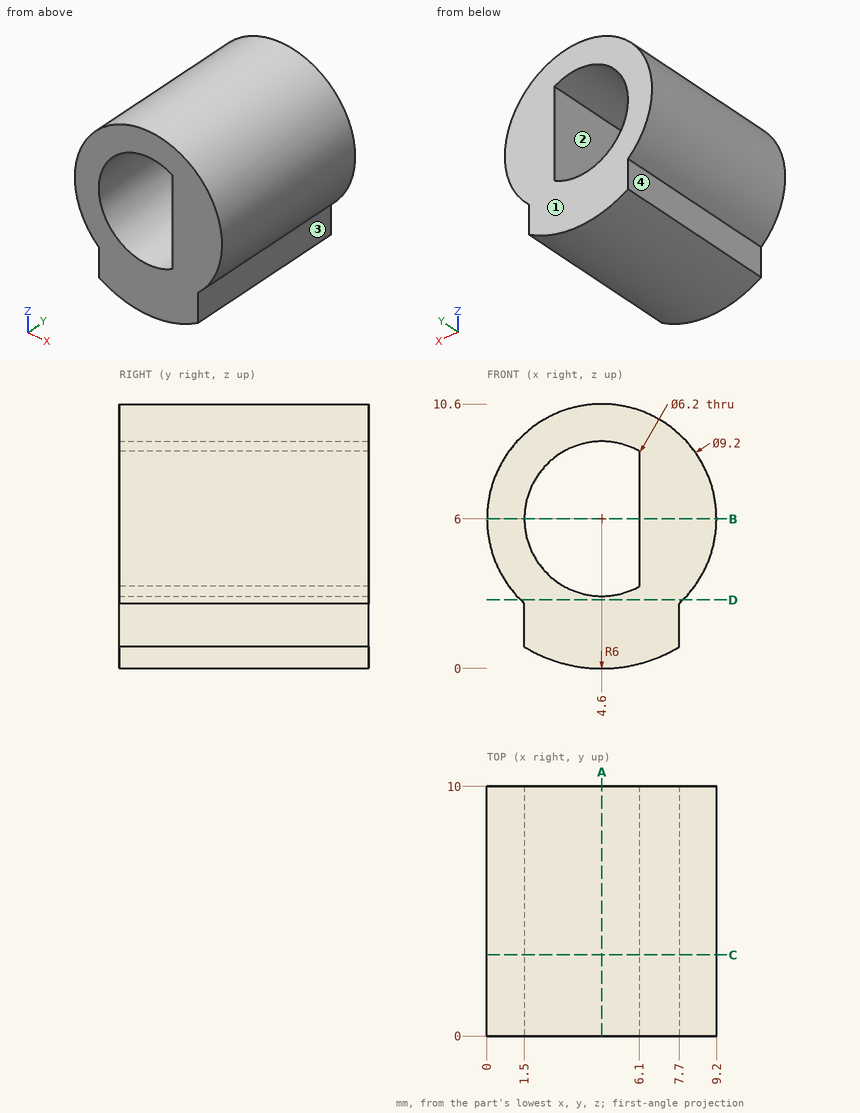
Can you work these out from the drawing? Everything is in mm from the part's minimum corner. Round coordinates to 2 decimals unless told otherwise and drop trailing zeros. Loops run counter-clockwise (first coordinate to the right, second up) from the corner with the lowest first, then second, coordinate; pieces in that order, holes last. Notation, with made-up numbers: (20, -37.5) - (29, -37.5) arc R32 ccw to (29, -9.5) - close; hole circle Ø5 at (-0.5, 49). An arc over 180 degrees is marked (long way). One line per question, with ' | ' between items. Start each with the question number.
Q1. I want a section at D-D (z = 2.75). Write out the boundary of the cut face in (x, y), then the cut area to 3 significant figures.
Q2. I want a section at B-B (z = 6). Write out the boundary of the cut face in (x, y), then the cut area to 3 significant figures.
Q3. Will these pins go through, and if not, where does the flat tip stop? pin 1 (0.5 mm diameter, centred on y = 4, z = 1.5, fed in from -X); pin 2 (6 mm diameter, centred on y = 8, z = 1, fed in from +X); pin 3 (0.5 mm diameter, centred on y = 3.5, z = 2, fed in from +X).
Q4. Please list where these lines run through material, in increasing order: line 1 (Z direction, x = 4.6, y = 5.5); line 2 (X direction, y = 7.25, z = 6); line 3 (X direction, y = 4.25, z = 4.5). Write a range as [from, to].
Q5. We'd pull the mould along X, two halves only. Please class the marked faces 1, 2, 3 and 4: +X half, -X half, draft (parallel to the pull), parting line (faces both ways), or undercut.
Q6. I want a section at C-C (y = 3.25). Write out the boundary of the cut face in (x, z).
Q7. I want a section at A-A (x = 4.6). Write out the boundary of the cut face in (y, z).
Response values:
1) outline: (1.34, 0) - (7.86, 0) - (7.86, 10) - (1.34, 10) - close | area: 65.1 mm²
2) outline: (0, 0) - (1.5, 0) - (1.5, 10) - (0, 10) - close; (6.1, 0) - (9.2, 0) - (9.2, 10) - (6.1, 10) - close | area: 46.0 mm²
3) pin 1: stops at x = 1.5 | pin 2: stops at x = 8.74 | pin 3: stops at x = 7.7
4) line 1: z = [0, 2.9], [9.1, 10.6] | line 2: x = [0, 1.5], [6.1, 9.2] | line 3: x = [0.25, 1.89], [6.1, 8.95]
5) face 1: draft | face 2: undercut | face 3: +X half | face 4: -X half
6) outline: (1.5, 0.86) arc R6 ccw to (7.7, 0.86) - (7.7, 2.6) arc R4.6 ccw (long way) to (1.5, 2.6) - close; hole (6.1, 3.29) - (6.1, 8.71) arc R3.1 ccw (long way) to start
7) outline: (0, 0) - (10, 0) - (10, 2.9) - (0, 2.9) - close; (0, 9.1) - (10, 9.1) - (10, 10.6) - (0, 10.6) - close
